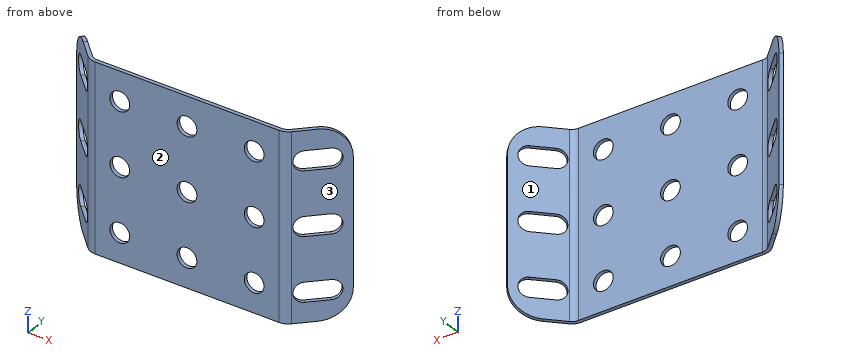
from build123d import *
from build123d.topology import SkipClean

# Parameters (mm, degrees)
ESTRUSIONE_SOTTILE1_DEPTH = 19
SCHIZZO2_R                = 2
TAGLIO_ESTRUSIONE2_DEPTH  = 10
TAGLIO_ESTRUSIONE3_DEPTH  = 10
RACCORDO1_R               = 6


with BuildPart() as part:
    # Schizzo1 → Estrusione-Sottile1 (new, symmetric)
    with BuildSketch(Plane.XY):
        with BuildLine():
            Line((-27.5, 8), (-20.085786438, 0.585786438))
            ThreePointArc((-20.085786438, 0.585786438), (-19.43693974, 0.152240935), (-18.671572875, 0))
            Line((-18.671572875, 0), (0, 0))
            Line((0, 0), (0, -0.75))
            Line((0, -0.75), (-18.671572875, -0.75))
            ThreePointArc((-18.671572875, -0.75), (-19.723952314, -0.540668714), (-20.616116524, 0.055456352))
            Line((-20.616116524, 0.055456352), (-28.030330086, 7.469669914))
            Line((-28.030330086, 7.469669914), (-27.5, 8))
        make_face()
    extrude(amount=ESTRUSIONE_SOTTILE1_DEPTH, both=True)

    # Schizzo2 → Taglio-Estrusione2 (cut)
    with BuildSketch(Plane.XZ.offset(0.75)):
        with Locations(Location((-13.616116524, -13, 0), (0, 0, 270))):
            Circle(SCHIZZO2_R)
        with Locations((0, -13)):
            Circle(SCHIZZO2_R)
        with Locations(Location((-13.616116524, 0, 0), (0, 0, 270))):
            Circle(SCHIZZO2_R)
        Circle(SCHIZZO2_R)
        with Locations((0, 13)):
            Circle(SCHIZZO2_R)
        with Locations(Location((-13.616116524, 13, 0), (0, 0, 270))):
            Circle(SCHIZZO2_R)
    extrude(amount=-TAGLIO_ESTRUSIONE2_DEPTH, mode=Mode.SUBTRACT)

    # Schizzo3 → Taglio-Estrusione3 (cut)
    with BuildSketch(Plane(origin=(-9.75, -9.75, 0), x_dir=(0, 0, -1), z_dir=(0.7071067811865487, 0.7071067811865465, 0))):
        with BuildLine():
            Line((-11, 21.352290732), (-11, 16.852290732))
            ThreePointArc((-11, 16.852290732), (-13, 14.852290732), (-15, 16.852290732))
            Line((-15, 16.852290732), (-15, 21.352290732))
            ThreePointArc((-15, 21.352290732), (-13, 23.352290732), (-11, 21.352290732))
        make_face()
        with BuildLine():
            Line((2, 21.352290732), (2, 16.852290732))
            ThreePointArc((2, 16.852290732), (0, 14.852290732), (-2, 16.852290732))
            Line((-2, 16.852290732), (-2, 21.352290732))
            ThreePointArc((-2, 21.352290732), (0, 23.352290732), (2, 21.352290732))
        make_face()
        with BuildLine():
            Line((11, 16.852290732), (11, 21.352290732))
            ThreePointArc((11, 21.352290732), (13, 23.352290732), (15, 21.352290732))
            Line((15, 21.352290732), (15, 16.852290732))
            ThreePointArc((15, 16.852290732), (13, 14.852290732), (11, 16.852290732))
        make_face()
    extrude(amount=-TAGLIO_ESTRUSIONE3_DEPTH, mode=Mode.SUBTRACT)

    # Raccordo1
    raccordo1_edges = [part.edges().sort_by_distance(p)[0] for p in [
        (-27.765165043, 7.734834957, 19),
        (-27.765165043, 7.734834957, -19),
    ]]
    fillet(raccordo1_edges, radius=RACCORDO1_R)

    # Specchia1: part across plane


with BuildPart() as part_1:
    with SkipClean():  # the faces are left unmerged after this step: merging them gives an invalid solid
        add(part.part)
        add(part.part.mirror(Plane(origin=(0, 0, 19), x_dir=(0, 0, 1), z_dir=(1, 0, 0))))


solid = part_1.part
For this review, take the finished solid that the model builds, in its own axes (mm). Face numbers are marked on the shaded views. Round coordinates to 2 decimals unless told otherwise and drop trailing zeros. Loops run counter-clockwise (first coordinate to the right, second up) from the corner with the lowest first, then second, coordinate; pieces in that order, holes last. Notation, with made-up numbers: (82, 36) - (105, 36) arc R22 cw to (105, 72) - close; hole circle Ø4 at (-27, 11.5). An arc over 180 degrees is marked (long way). Answer as CSV lines item,"result".
(1) Consider section D-D on x = 15. Give the boundary of the cut face in (y, z), then the cut area to 3 significant figures.
Checked values:
outline,"(-0.75, -19) - (0, -19) - (0, -14.44) - (-0.75, -14.44) - close; (-0.75, -11.56) - (0, -11.56) - (0, -1.44) - (-0.75, -1.44) - close; (-0.75, 1.44) - (0, 1.44) - (0, 11.56) - (-0.75, 11.56) - close; (-0.75, 14.44) - (0, 14.44) - (0, 19) - (-0.75, 19) - close"
area,"22.0 mm2"
(2) Consider section B-B on z = 5. Give the boundary of the cut face in (x, y), then the cut area to 3 significant figures.
Checked values:
outline,"(-28.03, 7.47) - (-20.62, 0.06) arc R2.75 ccw to (-18.67, -0.75) - (18.67, -0.75) arc R2.75 ccw to (20.62, 0.06) - (28.03, 7.47) - (27.5, 8) - (20.09, 0.59) arc R2 cw to (18.67, 0) - (-18.67, 0) arc R2 cw to (-20.09, 0.59) - (-27.5, 8) - close"
area,"46.5 mm2"
(3) Consider section A-A on x = 0. Give the boundary of the cut face in (y, z).
Checked values:
outline,"(-0.75, -19) - (0, -19) - (0, -15) - (-0.75, -15) - close; (-0.75, -11) - (0, -11) - (0, -2) - (-0.75, -2) - close; (-0.75, 2) - (0, 2) - (0, 11) - (-0.75, 11) - close; (-0.75, 15) - (0, 15) - (0, 19) - (-0.75, 19) - close"
(4) Wall thickness on line 1 (Z direction, x = 0, y = -0.2); line 2 (X direction, y = -0.25, z = -13); line 3 (X direction, y = -0.45, z = 0): over which ranges is each line inside the solid? List them lowest first.
Checked values:
line 1,"z = -19 to -15, -11 to -2, 2 to 11, 15 to 19"
line 2,"x = -20.25 to -15.62, -11.62 to -2, 2 to 11.62, 15.62 to 20.25"
line 3,"x = -19.92 to -15.62, -11.62 to -2, 2 to 11.62, 15.62 to 19.92"
(5) Insertion check: P1, Ø2.5, axis at x = 13.62, z = -13, coming from the -Y side; P2, Ø3, axis at y = 3.5, z = 4, coming from the +X side; P3, Ø5, axis at x = 0, z = 0, coming from the +Y side; P4, Ø3, axis at y = 4, z = -4, coming from the +X side. Each pin has a flat end and moves straight along its axis. Give the tip position at first contact, or say it passes through.
Checked values:
P1,"passes through"
P2,"stops at x = 25.56"
P3,"stops at y = 0"
P4,"stops at x = 26.06"
(6) Consider section C-C on z = 0. Give the number of separate pieces and of enclosed holes in the cut face, then the cut area to 3 significant figures.
Checked values:
separate pieces,"6"
enclosed holes,"0"
area,"24.8 mm2"
(7) Mouldability with a two-part tool opening along X and no side actions: class the marked faces 1, 2 and 3 as +X half, -X half, draft (parallel to the pull), parting line (faces both ways), or undercut.
Checked values:
face 1,"undercut"
face 2,"draft"
face 3,"+X half"
